Autodesk Inventor part; units mm, degrees
ref_plane "YZ Plane" through (0, 0, 0) normal (1, 0, 0) x (0, 1, 0)
ref_plane "XZ Plane" through (0, 0, 0) normal (0, 1, 0) x (-1, 0, 0)
ref_plane "XY Plane" through (0, 0, 0) normal (0, 0, 1) x (1, 0, 0)
sketch "Sketch1" plane through (0, 0, 0) normal (0, 0, 1) x (1, 0, 0)
  line L0 (22.86, 101.6) -> (22.86, 12.7)
  line L1 (22.86, 101.6) -> (0, 101.6) construction
  line L2 (0, 101.6) -> (0, 12.7)
  line L3 (0, 12.7) -> (22.86, 12.7)
  line L4 (0, 101.6) -> (0, 122.1962)
  line L5 (0, 122.1962) -> (10.16, 122.1962) construction
  line L6 (10.16, 122.1962) -> (0, 122.1962)
  line L7 (0, 122.1962) -> (0, 134.8962)
  line L8 (0, 134.8962) -> (10.16, 134.8962)
  line L9 (10.16, 134.8962) -> (10.16, 122.1962)
  line L10 (0, 12.7) -> (0, 0)
  arc A0 (0, 0) -> (22.86, 12.7) centre (0, 26.924) ccw
  line L11 (0, 0) -> (22.86, 0) construction
  line L12 (22.86, 0) -> (22.86, 12.7) construction
  arc A1 (22.86, 101.6) -> (10.16, 122.1962) centre (-0.1909, 101.6) ccw
  point P0 (0, 122.1962)
  dimension "d0" = 88.9
  dimension "d1" = 22.86
  dimension "d3" = 10.16
  dimension "d4" = 12.7
  dimension "d5" = 12.7
revolve "Revolution1" add sketch "Sketch1" angle 360 about axis through (0, 101.6, 0) along (0, -1, 0)
fillet "Fillet1" radius 6 1 edges at (-22.86, 12.7, 0)
fillet "Fillet2" radius 3.175 1 edges at (-10.16, 122.1962, 0)
sketch "Sketch2" plane through (0, 134.8962, 0) normal (0, 1, 0) x (1, 0, 0)
  circle A0 centre (0, 0) radius 10.16
  circle A1 centre (0, 0) radius 6.35
  point P0 (0, 0)
  dimension "d9" = 12.7
extrude "Extrusion1" cut sketch "Sketch2" against normal blind 25.4 contours A1
sketch "Sketch3" plane through (0, 109.4962, 0) normal (0, 1, 0) x (1, 0, 0)
  circle A0 centre (0, 0) radius 15.875
  dimension "d12" = 31.75
extrude "Extrusion2" cut sketch "Sketch3" against normal blind 101.6
fillet "Fillet3" radius 6.35 2 edges at (-15.875, 109.4962, 0) (-15.875, 7.8962, 0)
fillet "Fillet4" radius 1 1 edges at (-10.16, 134.8962, 0)
properties part number "CO2Cartridge16g"
Geometry check sheet. Reference: the model listing, model coordinates, mm. A direction names the side the tool comes from. Give positions to 0.01 mm unless a question says otherwise; leave off trailing zeros. Order: outer loops, then holes, each group sorted by start corner. A loop starts at its lowest first (then second) coordinate and runs counter-clockwise, first axis right, second up. Notation, with made-up numbers: (-24, -12) - (4, -12) arc R17 ccw to (4, 6) - close; hole circle Ø11 at (23, -32). An arc over 180 degrees is marked (long way). Answer as a JSON object with one key per item and string values.
(1) Depth check by flat-ended pin: pin 1 Ø3 at (y, z) = (36, -3.5) entering from +X; pin 2 Ø4 at (x, z) = (-14.5, 9) entering from +Y; pin 3 Ø6 at (x, z) = (-5.5, 12.5) entering from +Y. Enter the tip coordinate at first touch or a pass-through.
Report:
{"pin 1": "x = 22.77", "pin 2": "y = 118.88", "pin 3": "y = 122.36"}
(2) Cross-section at A-A (y = 92.5). Record the cut outline in (x, z) (3 decimals).
Report:
{"outline": "circle Ø45.72 at (0, 0); hole circle Ø31.75 at (0, 0)"}
(3) Tool access check on faces 4 (the cylindrical face through (-1.323, 128.914, 10.074)), 5 (the flat face through (0, 7.896, 0)). Record the directions out of +Z, -Z, +X, -X, +Y, -Y that give a thin tool (end or side, any length) a straight path to the whole face; none if there is none.
Report:
{"face 4": "+Y", "face 5": "none"}
(4) Draft check along Z on faces 1 (the cylindrical face through (21.804, 57.457, 6.867)), 2 (the flat face through (1.91, 134.896, 6.23)), 3 (the flat face through (6.2, 109.496, 2)). Enter one of: released by +Z, released by -Z, zero draft, split by the parting line, or undercut.
Report:
{"face 1": "split by the parting line", "face 2": "zero draft", "face 3": "undercut"}
(5) Material ranges on line 1 (Z direction, x = 0, y = 74) (3 decimals); line 2 (X direction, y = 115.5, z = 0), recorded low to high.
Report:
{"line 1": "-22.86 to -15.875, 15.875 to 22.86", "line 2": "-18.2 to -6.35, 6.35 to 18.2"}
